The listing builds one solid part. Answer for the finished solid, in the listing's coordinates (mm). A direction names the side the tool comes from. Round coordinates to 2 decimals unless told otherwise and drop trailing zeros. Write each loop counter-clockwise with the first axis right and the second up, starting at its lowest first coordinate (ties: lowest second). Pieces come first, ordered by that corner, then holes. Notation, with made-up numbers: (53.5, 56.5) - (64.5, 56.5) arc R7 ccw to (64.5, 60.5) - close; hole circle Ø8 at (-23.5, 6). An arc over 180 degrees is marked (long way). Answer in a Markdown table with one row per item.
from build123d import *

# Parameters (mm, degrees)
F3_DEPTH = 2


with BuildPart() as f1:
    # F0 (on Front) → F1 (revolve)
    with BuildSketch(Plane.XZ):
        Polygon((4, 0), (0, 0), (0, -18), (2, -18), (2, -2), align=None)
    revolve(axis=Axis((0, 0, -9), (0, 0, 1)))

    # F2 (on face) → F3 (cut)
    with BuildSketch(Plane.XY):
        Polygon((0.721688, 1.25), (-0.721688, 1.25), (-1.443376, 0), (-0.721688, -1.25), (0.721688, -1.25), (1.443376, 0), align=None)
    extrude(amount=-F3_DEPTH, mode=Mode.SUBTRACT)


solid = f1.part
(1) Flat-ended cylindrical pins translate along their axes: pin 1 (1.5 mm diameter, centred on y = 0.5, z = -8, fed in from +X); pin 2 (1.2 mm diameter, centred on x = 0, z = -1, fed in from -Y); pin 3 (0.8 mm diameter, centred on x = 0, y = 0, fed in from +Z). Find the tip coordinate at first contact, or state that the pin passes through.
Checked values:
| item | result |
|---|---|
| pin 1 | stops at x = 2 |
| pin 2 | stops at y = -3.6 |
| pin 3 | stops at z = -2 |
(2) For faces 4 (the flat face through (2, 0, 0)), 5 (the flat face through (0, 0, -2)), determine the directions among +Z, -Z, +X, -X, +Y, -Y from which every point of the face is accessible in a straight line to the end or side of a thin tool.
Checked values:
| item | result |
|---|---|
| face 4 | +Z, +X, -X, +Y, -Y |
| face 5 | +Z |
(3) Find the intervals of material crossed by line 1 (Z direction, x = -1, y = 0.5); line 2 (Y direction, x = 0, z = -9.25); line 3 (Y direction, x = 0.5, z = -16), in increasing order.
Checked values:
| item | result |
|---|---|
| line 1 | z = -18 to -2 |
| line 2 | y = -2 to 2 |
| line 3 | y = -1.94 to 1.94 |
(4) Section B-B (z = -6.5) is taken. Give the vertices of the cut face in (x, y), and give its area (3 significant figures).
Checked values:
| item | result |
|---|---|
| outline | circle Ø4 at (0, 0) |
| area | 12.6 mm2 |
(5) Section A-A (x = 0) is taken. Give the vertices of the cut face in (y, z), and give its area (3 significant figures).
Checked values:
| item | result |
|---|---|
| outline | (-4, 0) - (-2, -2) - (-2, -18) - (2, -18) - (2, -2) - (4, 0) - (1.25, 0) - (1.25, -2) - (-1.25, -2) - (-1.25, 0) - close |
| area | 71.0 mm2 |
(6) For a pull along X with two mould halves and no side action, classify faces 1 (the flat face through (0, 1.25, -1)), 2 (the cylindrical face through (0, -2, -10)), 3 (the flat face through (0, 0, -18)) as pulls with the +X half, pulls with the -X half, needs draft (parallel to the pull), parting line crosses it, or undercut.
Checked values:
| item | result |
|---|---|
| face 1 | undercut |
| face 2 | parting line crosses it |
| face 3 | needs draft |
